Here's how the part is built. I have some questions about the finished solid (model axes, mm). Face numbers are marked on the shaded views. A direction names the side the tool comes from. Round coordinates to 2 decimals unless told otherwise and drop trailing zeros. Write each loop counter-clockwise with the first axis right and the second up, starting at its lowest first coordinate (ties: lowest second). Pieces come first, ordered by that corner, then holes. Notation, with made-up numbers: (16, 27.5) - (56, 27.5) arc R20 ccw to (56, 42.5) - close; hole circle Ø4 at (-28, -30). An arc over 180 degrees is marked (long way). One line per question, with ' | ' between items. Start each with the question number.
(1) For the marked faces 1, 2 and 3, which set-ups out of +Z, -Z, +X, -X, +Y, -Y let a thin tool reach every point of the face, with its end or its side?
(2) Will these pins go through, and if not, where does the flat tip stop? pin 1 (3 mm diameter, centred on x = 13, y = 26, fed in from -Z); pin 2 (3 mm diameter, centred on y = 29, z = 4, fed in from +X) (3 decimals); pin 3 (3 mm diameter, centred on x = 19, z = -1, fed in from +Y); pin 4 (10 mm diameter, centred on x = 22, y = 26, fed in from -Z).
(3) If I drill on L1, parallel to Y at x = 20, z = -0.25; L2, parallel to X at y = 17.5, z = -0.5; L3, parallel to Z at x = 16, y = 15, over which ranges is the centre line in solid material (lowest first)?
(4) Thinking about a two-plate mould opening in X: for the marked faces 4, 5, 6 and 7, which applies, pulls with the +X half, pulls with the -X half, needs draft (parallel to the pull), parting line crosses it, or undercut?
(5) Imagine slicing it at A-A (z = -1.25). Write out the boundary of the cut face in (x, y) (3 decimals).
(6) Imagine slicing it at C-C (x = 22.5). Write out the boundary of the cut face in (y, z), plus the area to 3 significant figures.
(7) Imagine slicing it at B-B (z = 2.5). Write out the boundary of the cut face in (x, y) (1 decimal).
(8) Imagine slicing it at D-D (y = 12). Write out the boundary of the cut face in (x, z).
Autodesk Inventor part; units mm, degrees
ref_plane "YZ Plane" through (0, 0, 0) normal (1, 0, 0) x (0, 1, 0)
ref_plane "XZ Plane" through (0, 0, 0) normal (0, 1, 0) x (-1, 0, 0)
ref_plane "XY Plane" through (0, 0, 0) normal (0, 0, 1) x (1, 0, 0)
sketch "Sketch1" plane through (0, 0, 0) normal (0, 0, 1) x (1, 0, 0)
  line L0 (0, 0) -> (0, 22.1234)
  line L1 (0, 22.1234) -> (10.795, 22.1234)
  line L2 (10.795, 22.1234) -> (10.795, 31.6484)
  line L3 (10.795, 31.6484) -> (19.685, 31.6484)
  line L4 (19.685, 31.6484) -> (19.685, 22.1234)
  line L5 (19.685, 22.1234) -> (30.48, 22.1234)
  line L6 (30.48, 22.1234) -> (30.48, 0)
  line L7 (30.48, 0) -> (0, 0)
  dimension "d0" = 10.795
  dimension "d1" = 9.525
  dimension "d2" = 8.89
  dimension "d3" = 10.795
  dimension "d17" = 31.6484
extrude "Extrusion1" add sketch "Sketch1" along normal blind 6.2484
sketch "Sketch2" plane through (19.685, 22.1234, 0) normal (1, 0, 0) x (0, 0, -1)
  circle A0 centre (-3.1242, 6.4008) radius 1.8542
  line L0 (0, 9.525) -> (-6.2484, 9.525)
  line L1 (-3.1242, 9.525) -> (-3.1242, 0) construction
  line L2 (0, 0) -> (-6.2484, 0)
  point P0 (0, -22.1234)
  dimension "d7" = 3.7084
  dimension "d8" = 3.1242
extrude "Extrusion2" cut sketch "Sketch2" against normal through all
fillet "Fillet1" radius 3.1242 2 edges at (15.24, 31.6484, 6.2484) (15.24, 31.6484, 0)
chamfer "Chamfer1" distance 1.905 angle 45 6 edges at (19.685, 22.1234, 3.1242) (10.795, 22.1234, 3.1242) (30.48, 22.1234, 3.1242) (0, 22.1234, 3.1242) (30.48, 0, 3.1242) (0, 0, 3.1242)
sketch "Sketch4" plane through (0, 0, 0) normal (0, 0, -1) x (-1, 0, 0)
  line L0 (-21.59, 22.1234) -> (-8.89, 22.1234)
  line L1 (-1.905, 22.1234) -> (-8.89, 22.1234)
  line L2 (-1.905, 22.1234) -> (0, 20.2184)
  line L3 (0, 1.905) -> (0, 20.2184)
  line L4 (0, 1.905) -> (-1.905, 0)
  line L5 (-28.575, 0) -> (-1.905, 0)
  line L6 (-28.575, 0) -> (-30.48, 1.905)
  line L7 (-30.48, 20.2184) -> (-30.48, 1.905)
  line L8 (-30.48, 20.2184) -> (-28.575, 22.1234)
  line L9 (-21.59, 22.1234) -> (-28.575, 22.1234)
  line L10 (-28.0489, 20.8534) -> (-29.21, 19.6923)
  line L11 (-29.21, 19.6923) -> (-29.21, 2.4311)
  line L12 (-29.21, 2.4311) -> (-28.0489, 1.27)
  line L13 (-28.0489, 1.27) -> (-2.4311, 1.27)
  line L14 (-2.4311, 1.27) -> (-1.27, 2.4311)
  line L15 (-1.27, 2.4311) -> (-1.27, 19.6923)
  line L16 (-1.27, 19.6923) -> (-2.4311, 20.8534)
  line L17 (-2.4311, 20.8534) -> (-8.89, 20.8534)
  line L18 (-8.89, 20.8534) -> (-21.59, 20.8534)
  line L19 (-21.59, 20.8534) -> (-28.0489, 20.8534)
  line L20 (-29.21, 3.175) -> (-1.27, 3.175)
  point P0 (0, 0)
  point P1 (-29.21, 3.81)
  point P2 (-30.48, 3.81)
  point P3 (-1.27, 3.81)
  point P4 (0, 3.81)
  dimension "d18" = 1.27
  dimension "d19" = 3.175
extrude "Extrusion3" add sketch "Sketch4" along normal blind 2.794
properties part number "SDCardCover"
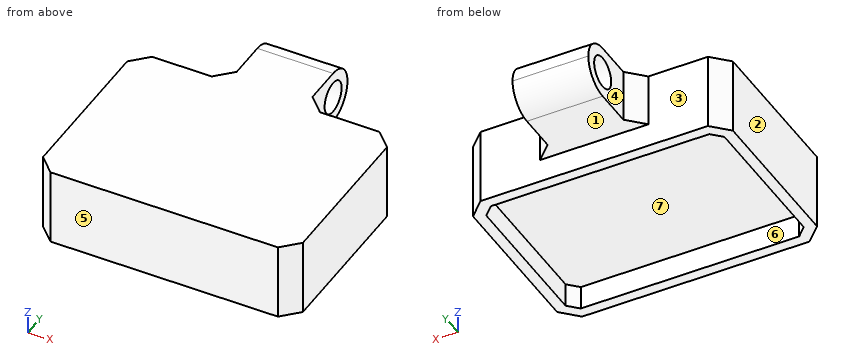
Check sheet entries:
1) face 1: -Z, +X, -X, +Y | face 2: +Z, -Z, -X, +Y, -Y | face 3: -Z, +Y
2) pin 1: z = 0 | pin 2: x = 19.685 | pin 3: y = 30.22 | pin 4: z = -2.79
3) L1: 0 to 1.27, 20.85 to 22.12 | L2: 0 to 1.27, 29.21 to 30.48 | L3: 0 to 6.25
4) face 4: pulls with the -X half | face 5: needs draft | face 6: undercut | face 7: undercut
5) outline: (0, 1.905) - (1.905, 0) - (28.575, 0) - (30.48, 1.905) - (30.48, 20.218) - (28.575, 22.123) - (1.905, 22.123) - (0, 20.218) - close; hole (1.27, 2.431) - (2.431, 1.27) - (28.049, 1.27) - (29.21, 2.431) - (29.21, 19.692) - (28.049, 20.853) - (2.431, 20.853) - (1.27, 19.692) - close
6) outline: (0, -2.79) - (1.27, -2.79) - (1.27, 0) - (20.85, 0) - (20.85, -2.79) - (22.12, -2.79) - (22.12, 6.25) - (0, 6.25) - close | area: 145 mm^2
7) outline: (0, 1.9) - (1.9, 0) - (28.6, 0) - (30.5, 1.9) - (30.5, 20.2) - (28.6, 22.1) - (21.6, 22.1) - (19.7, 24) - (19.7, 26.8) - (10.8, 26.8) - (10.8, 24) - (8.9, 22.1) - (1.9, 22.1) - (0, 20.2) - close; (10.8, 30.3) - (19.7, 30.3) - (19.7, 31.6) - (10.8, 31.6) - close
8) outline: (0, -2.79) - (1.27, -2.79) - (1.27, 0) - (29.21, 0) - (29.21, -2.79) - (30.48, -2.79) - (30.48, 6.25) - (0, 6.25) - close
